Could you check a few things on this model? Use its own coordinates, in mm. A direction names the side the tool comes from. Give positions to 0.01 mm unless a question says otherwise; leave off trailing zeros. Order: outer loops, then holes, each group sorted by start corner. A loop starts at its lowest first (then second) coordinate and runs counter-clockwise, first axis right, second up. Notation, with made-up numbers: (-21, 25.25) -> (13, 25.25) arc R30 cw to (13, 51.25) -> close; hole circle Ø11 at (-5, 78.5). An arc over 180 degrees is marked (long way). Write each question's results on one line, items separated by ' | '.
```python
from build123d import *

# Parameters (mm, degrees)
SKETCH1_W           = 190
SKETCH1_H           = 190
BOSS_EXTRUDE1_DEPTH = 10
CUT_EXTRUDE1_DEPTH  = 5
SKETCH3_W           = 60
SKETCH3_H           = 60
CUT_EXTRUDE2_DEPTH  = 139.021737418
CUT_EXTRUDE3_DEPTH  = 3
SKETCH8_W           = 40.8
SKETCH8_H           = 12.294985481
CUT_EXTRUDE4_DEPTH  = 2.6
CUT_EXTRUDE5_DEPTH  = 7
FILLET1_R           = 3
SKETCH10_W          = 3.1
SKETCH10_H          = 5.2
CUT_EXTRUDE6_DEPTH  = 15
FILLET2_R           = 1
SKETCH11_W          = 3.1
SKETCH11_H          = 5.2
CUT_EXTRUDE7_DEPTH  = 15
FILLET3_R           = 1
FILLET4_R           = 4
SKETCH12_W          = 4
SKETCH12_H          = 5.2
CUT_EXTRUDE8_DEPTH  = 2
SKETCH13_W          = 3
SKETCH13_H          = 5.2
CUT_EXTRUDE9_DEPTH  = 6
SKETCH14_W          = 3
SKETCH14_H          = 10
BOSS_EXTRUDE2_DEPTH = 7
SKETCH16_W          = 3.2
SKETCH16_H          = 5
CUT_EXTRUDE10_DEPTH = 6
FILLET5_R           = 1
SKETCH17_W          = 131.159114754
SKETCH17_H          = 131.95401848
CUT_EXTRUDE11_DEPTH = 2.1
CUT_EXTRUDE12_DEPTH = 2


with BuildPart() as part:
    # Sketch1 → Boss-Extrude1 (new body)
    with BuildSketch(Plane(origin=(0, 0, 0), x_dir=(0, 0, -1), z_dir=(1, 0, 0))):
        with Locations((-5, 0)):
            Rectangle(SKETCH1_W, SKETCH1_H)
    extrude(amount=BOSS_EXTRUDE1_DEPTH)

    # Sketch2 → Cut-Extrude1 (cut)
    with BuildSketch(Plane.ZY):
        Polygon((36.5, -36.5), (36.5, 36.5), (25.709845909, 36.5), (5.209845909, 45.5), (-5.209845909, 45.5), (-25.709845909, 36.5), (-36.5, 36.5), (-36.5, -36.5), align=None)
    extrude(amount=-CUT_EXTRUDE1_DEPTH, mode=Mode.SUBTRACT)

    # Sketch3 → Cut-Extrude2 (cut, through all)
    with BuildSketch(Plane.ZY.offset(-5)):
        Rectangle(SKETCH3_W, SKETCH3_H)
    extrude(amount=-CUT_EXTRUDE2_DEPTH, mode=Mode.SUBTRACT)

    # Sketch4 → Cut-Extrude3 (cut)
    with BuildSketch(Plane(origin=(10, 0, 0), x_dir=(0, 0, -1), z_dir=(1, 0, 0))):
        with BuildLine():
            Line((35, 29.999999003), (35, -35.000000997))
            Line((35, -35.000000997), (35, -36.000000997))
            Line((35, -36.000000997), (14.142135624, -35.000000997))
            ThreePointArc((14.142135624, -35.000000997), (8.484611805, -38.299622231), (8.570991287, -44.848485845))
            ThreePointArc((8.570991287, -44.848485845), (0, -60.000000997), (-8.570991287, -44.848485845))
            ThreePointArc((-8.570991287, -44.848485845), (-8.484611805, -38.299622231), (-14.142135624, -35.000000997))
            Line((-14.142135624, -35.000000997), (-36, -36.000000997))
            Line((-36, -36.000000997), (-35.000001658, -14.142137383))
            ThreePointArc((-35.000001658, -14.142137383), (-38.29962223, -8.484613177), (-44.848485854, -8.570991891))
            ThreePointArc((-44.848485854, -8.570991891), (-60, 1.173e-06), (-44.848483843, 8.570990683))
            ThreePointArc((-44.848483843, 8.570990683), (-38.29962024, 8.484610433), (-34.999998342, 14.142133865))
            Line((-34.999998342, 14.142133865), (-36, 34.999999003))
            Line((-36, 34.999999003), (-35, 34.999999003))
            Line((-35, 34.999999003), (30, 34.999999003))
            ThreePointArc((30, 34.999999003), (33.535533906, 33.535532909), (35, 29.999999003))
        make_face()
    extrude(amount=-CUT_EXTRUDE3_DEPTH, mode=Mode.SUBTRACT)

    # Sketch8 → Cut-Extrude4 (cut)
    with BuildSketch(Plane.ZY):
        with Locations((0, 92.547492741)):
            Rectangle(SKETCH8_W, SKETCH8_H)
    extrude(amount=-CUT_EXTRUDE4_DEPTH, mode=Mode.SUBTRACT)

    # Sketch9 → Cut-Extrude5 (cut)
    # profile 1 of 2: a face of its own
    with BuildSketch(Plane.ZY):
        Polygon((-25.4, 90), (-85, 90), (-85, -90), (95, -90), (95, 90), (25.4, 90), (25.4, 81.4), (-25.4, 81.4), align=None)
        Polygon((-41.5, -41.5), (-41.5, 41.5), (-19.296204392, 41.5), (-5.629537726, 47.5), (5.629537726, 47.5), (19.296204392, 41.5), (41.5, 41.5), (41.5, 12.5), (61.5, 12.5), (61.5, -12.5), (41.5, -12.5), (41.5, -41.5), (12.5, -41.5), (12.5, -61.5), (-12.5, -61.5), (-12.5, -41.5), align=None, mode=Mode.SUBTRACT)
    # profile 2 of 2: a face of its own
    with BuildSketch(Plane.ZY):
        Polygon((-5.629537726, 47.5), (5.629537726, 47.5), (5.209845909, 45.5), (-5.209845909, 45.5), align=None)
    extrude(amount=-CUT_EXTRUDE5_DEPTH, mode=Mode.SUBTRACT)

    # Fillet1
    fillet1_edges = [part.edges().sort_by_distance(p)[0] for p in [
        (10, 95, 5),
        (10, 0, 100),
        (5, 95, 100),
        (5, -95, 100),
        (10, -95, 5),
    ]]
    fillet(fillet1_edges, radius=FILLET1_R)

    # Sketch10 → Cut-Extrude6 (cut)
    with BuildSketch(Plane.XZ.offset(61.5)):
        with Locations((4.25, 0)):
            Rectangle(SKETCH10_W, SKETCH10_H)
    extrude(amount=-CUT_EXTRUDE6_DEPTH, mode=Mode.SUBTRACT)

    # Fillet2
    fillet2_edges = [part.edges().sort_by_distance(p)[0] for p in [
        (2.7, -61.5, 0),
        (4.25, -61.5, -2.6),
        (5.8, -61.5, 0),
        (4.25, -61.5, 2.6),
    ]]
    fillet(fillet2_edges, radius=FILLET2_R)

    # Sketch11 → Cut-Extrude7 (cut)
    with BuildSketch(Plane.XY.offset(61.5)):
        with Locations((4.25, 0)):
            Rectangle(SKETCH11_W, SKETCH11_H)
    extrude(amount=-CUT_EXTRUDE7_DEPTH, mode=Mode.SUBTRACT)

    # Fillet3
    fillet3_edges = [part.edges().sort_by_distance(p)[0] for p in [
        (2.7, 0, 61.5),
        (4.25, -2.6, 61.5),
        (5.8, 0, 61.5),
        (4.25, 2.6, 61.5),
    ]]
    fillet(fillet3_edges, radius=FILLET3_R)

    # Fillet4
    fillet4_edges = [part.edges().sort_by_distance(p)[0] for p in [
        (3.5, -61.5, -12.5),
        (3.5, -61.5, 12.5),
        (3.5, -12.5, 61.5),
        (3.5, 12.5, 61.5),
    ]]
    fillet(fillet4_edges, radius=FILLET4_R)

    # Sketch12 → Cut-Extrude8 (cut)
    with BuildSketch(Plane.ZY):
        with Locations((-87, -82.4)):
            Rectangle(SKETCH12_W, SKETCH12_H)
    extrude(amount=-CUT_EXTRUDE8_DEPTH, mode=Mode.SUBTRACT)

    # Sketch13 → Cut-Extrude9 (cut)
    with BuildSketch(Plane.ZY.offset(-2)):
        with Locations((-87.5, -82.4)):
            Rectangle(SKETCH13_W, SKETCH13_H)
    extrude(amount=-CUT_EXTRUDE9_DEPTH, mode=Mode.SUBTRACT)

    # Sketch14 → Boss-Extrude2 (add)
    with BuildSketch(Plane.ZY.offset(-7)):
        with Locations((93.5, -82.4)):
            Rectangle(SKETCH14_W, SKETCH14_H)
    extrude(amount=BOSS_EXTRUDE2_DEPTH)

    # Sketch16 → Cut-Extrude10 (cut)
    with BuildSketch(Plane(origin=(0, 0, 92), x_dir=(-1, 0, 0), z_dir=(0, 0, -1))):
        with Locations((-2.8, -82.4)):
            Rectangle(SKETCH16_W, SKETCH16_H)
    extrude(amount=-CUT_EXTRUDE10_DEPTH, mode=Mode.SUBTRACT)

    # Fillet5
    fillet5_edges = [part.edges().sort_by_distance(p)[0] for p in [
        (4.4, -82.4, 92),
        (2.8, -84.9, 92),
        (2.8, -79.9, 92),
    ]]
    fillet(fillet5_edges, radius=FILLET5_R)

    # Sketch17 → Cut-Extrude11 (cut)
    with BuildSketch(Plane.ZY):
        Rectangle(SKETCH17_W, SKETCH17_H)
    extrude(amount=-CUT_EXTRUDE11_DEPTH, mode=Mode.SUBTRACT)

    # Sketch18 → Cut-Extrude12 (cut)
    with BuildSketch(Plane.ZY):
        Polygon((-23.4, 92), (-87, 92), (-87, -79.8), (-85, -79.8), (-85, 90), (-25.4, 90), (-25.4, 81.4), (25.4, 81.4), (25.4, 90), (95, 90), (95, -77.4), (97, -77.4), (97, 92), (23.4, 92), (23.4, 83.4), (-23.4, 83.4), align=None)
        Polygon((-85, -79.8), (-87, -79.8), (-87, -85), (-85, -85), (-85, -90), (95, -90), (95, -87.4), (92, -87.4), (92, -77.4), (95, -77.4), (95, 90), (25.4, 90), (25.4, 81.4), (-25.4, 81.4), (-25.4, 90), (-85, 90), align=None)
        Polygon((-85, -85), (-87, -85), (-87, -92), (97, -92), (97, -87.4), (95, -87.4), (95, -90), (-85, -90), align=None)
    extrude(amount=-CUT_EXTRUDE12_DEPTH, mode=Mode.SUBTRACT)


solid = part.part
```
Q1. I need wall thicknesses on line 1 along Z through (x, y) = (3.25, -47); line 2 along Z through (x, y) = (7.25, -36.5); line 3 along Y through (x, z) = (5.25, -72.5). Which ranges of each line are inside material? Lowest first, please.
Here are the results:
line 1: z = -90 to -85, -12.5 to -2.6, 2.6 to 12.5, 95 to 100 | line 2: z = -90 to -9.99, 9.99 to 99.99 | line 3: y = -95 to -90, 90 to 95
Q2. I'm going to push flat-ended pins straight in: pin 1 Ø12 at (y, z) = (-50, 0) entering from +X; pin 2 Ø4 at (y, z) = (51.5, 41) entering from -X; pin 3 Ø1.5 at (y, z) = (26, 30) entering from -X. Where does each tip first touch, or does it pass through?
Here are the results:
pin 1: stops at x = 7 | pin 2: stops at x = 7 | pin 3: stops at x = 5
Q3. For faces 4 (the flat face through (5, 32, -1)), 5 (the cylindrical face through (8.52, 8.44, 38.38)), 6 (the flat face through (5.8, -54, 0)), which set-ups out of +Z, -Z, +X, -X, +Y, -Y let a thin tool reach every point of the face, with its end or its side?
Here are the results:
face 4: -X | face 5: +X | face 6: none
Q4. Thinking about a two-plate mould opening in X: for faces 1 (the flat face through (4.4, -82, 95)), 2 (the flat face through (3, -95, 5)), 3 (the flat face through (2.6, 91, 0)), which applies, +X half, -X half, draft (parallel to the pull), parting line (faces both ways), or undercut?
Here are the results:
face 1: undercut | face 2: draft | face 3: -X half
Q5. Suppose I cut it at B-B on z = 50. Please give me the cut outline in (x, y).
Here are the results:
outline: (0, -95) -> (7, -95) arc R3 ccw to (10, -92) -> (10, -10) -> (7, -10) -> (7, 10) -> (10, 10) -> (10, 92) arc R3 ccw to (7, 95) -> (0, 95) -> (0, 92) -> (2, 92) -> (2, 90) -> (7, 90) -> (7, 12.5) -> (2.1, 12.5) -> (2.1, -12.5) -> (7, -12.5) -> (7, -90) -> (2, -90) -> (2, -92) -> (0, -92) -> close; hole (2.7, -2.6) -> (5.8, -2.6) -> (5.8, 2.6) -> (2.7, 2.6) -> close
Q6. Suppose I cut it at D-D on y = 69. Please give me the cut outline in (x, z), and give its area (3 significant figures).
Here are the results:
outline: (0, -90) -> (10, -90) -> (10, 97) arc R3 ccw to (7, 100) -> (0, 100) -> (0, 97) -> (2, 97) -> (2, 95) -> (7, 95) -> (7, -85) -> (2, -85) -> (2, -87) -> (0, -87) -> close | area: 630 mm²
